from build123d import *

# Parameters (mm, degrees)
SKETCH1_W           = 22
SKETCH1_H           = 40
SKETCH1_W_2         = 12
SKETCH1_H_2         = 30
BOSS_EXTRUDE1_DEPTH = 10
SKETCH2_R           = 1.5
CUT_EXTRUDE1_DEPTH  = 15


with BuildPart() as part:
    # Sketch1 → Boss-Extrude1 (new body)
    with BuildSketch(Plane.XY):
        with Locations((11, 20)):
            Rectangle(SKETCH1_W, SKETCH1_H)
        with Locations((11, 20)):
            Rectangle(SKETCH1_W_2, SKETCH1_H_2, mode=Mode.SUBTRACT)
    extrude(amount=BOSS_EXTRUDE1_DEPTH)

    # Sketch2 → Cut-Extrude1 (cut, symmetric)
    with BuildSketch(Plane(origin=(0, 0, 0), x_dir=(1, 0, 0), z_dir=(0, 1, 0))):
        with Locations(Location((11, -5, 0), (0, 0, 270))):
            Circle(SKETCH2_R)
    extrude(amount=CUT_EXTRUDE1_DEPTH, both=True, mode=Mode.SUBTRACT)


solid = part.part
Source: CAD feature listing. Evaluate the final solid. Frame: model axes, mm. A direction names the side the tool comes from. Coordinates: 2 decimals unless noted, no trailing zeros. Loops run counter-clockwise (first coordinate to the right, second up) from the corner with the lowest first, then second, coordinate; pieces in that order, holes last. Notation, with made-up numbers: (-13, 64) - (15, 64) arc R20 cw to (15, 86) - close; hole circle Ø6 at (10, 65). An arc over 180 degrees is marked (long way). Return JSON: item names as keys, results as strings.
Q1. Access query for faces 4 (the flat face through (5, 20, 5)), 5 (the cylindrical face through (10.425, 2.535, 6.386)), 6 (the flat face through (4, 20, 0)). Directions: +Z, -Z, +X, -X, +Y, -Y. A direction counts if a zero-diameter tool reaches every point of the face in a straight line with its end or side. Return the directions, or none.
Results:
{"face 4": "+Z, -Z", "face 5": "-Y", "face 6": "-Z, +X, -X, +Y, -Y"}
Q2. Section B-B, the plane y = 29.5. Return loops of the section in (x, z), plus the area to 3 significant figures.
Results:
{"outline": "(0, 0) - (5, 0) - (5, 10) - (0, 10) - close; (17, 0) - (22, 0) - (22, 10) - (17, 10) - close", "area": "100 mm2"}
Q3. Material intervals for line 1 along X through (y, z) = (3.3, 5); line 2 along Y through (x, z) = (9, 6); line 3 along X through (y, z) = (9.5, 7.5), sorted ascending.
Results:
{"line 1": "0 to 9.5, 12.5 to 22", "line 2": "0 to 5, 35 to 40", "line 3": "0 to 5, 17 to 22"}
Q4. Section C-C, the plane z = 2. Return loops of the section in (x, y), plus the area to 3 significant figures.
Results:
{"outline": "(0, 0) - (22, 0) - (22, 40) - (0, 40) - close; hole (5, 5) - (17, 5) - (17, 35) - (5, 35) - close", "area": "520 mm2"}
Q5. Mould query, pull axis X, two halves, no side actions, for faces 1 (the flat face through (11, 35, 5)), 2 (the flat face through (22, 20, 5)), 3 (the flat face through (11, 40, 5)). Classes: released by +X, released by -X, zero draft, split by the parting line, or undercut.
Results:
{"face 1": "undercut", "face 2": "released by +X", "face 3": "zero draft"}
Q6. Contact query for a flat-ended pin moving along its axis: P1, Ø2.5, axis at x = 11, z = 5, coming from the -Y side. Output: stop coordinate, or through.
Results:
{"P1": "y = 35"}
Q7. Section A-A, the plane x = 11. Return loops of the section in (y, z).
Results:
{"outline": "(0, 0) - (5, 0) - (5, 3.5) - (0, 3.5) - close; (0, 6.5) - (5, 6.5) - (5, 10) - (0, 10) - close; (35, 0) - (40, 0) - (40, 10) - (35, 10) - close"}
Q8. Section D-D, the plane z = 5. Return loops of the section in (x, y), plus the area to 3 significant figures.
Results:
{"outline": "(0, 0) - (9.5, 0) - (9.5, 5) - (5, 5) - (5, 35) - (17, 35) - (17, 5) - (12.5, 5) - (12.5, 0) - (22, 0) - (22, 40) - (0, 40) - close", "area": "505 mm2"}
